Geometry check sheet. Reference: the model listing, model coordinates, mm. Face numbers are marked on the shaded views. A direction names the side the tool comes from. Coordinates: 2 decimals unless noted, no trailing zeros. Loops run counter-clockwise (first coordinate to the right, second up) from the corner with the lowest first, then second, coordinate; pieces in that order, holes last. Notation, with made-up numbers: (-29, -7) - (10, -7) arc R20 ccw to (10, 23) - close; hole circle Ø10 at (23, -11.75). An arc over 180 degrees is marked (long way). One line per item, written item: value.
Autodesk Inventor part; units mm, degrees
ref_plane "to_bolt_XY" through (3, 9.5, 0) normal (1, 0, 0) x (0, 0, -1)
ref_plane "to_bolt_YZ" through (3, 9.5, 0) normal (0, 0, -1) x (0, 1, 0)
ref_plane "to_bolt_ZX" through (3, 9.5, 0) normal (0, 1, 0) x (1, 0, 0)
sketch "_____1" plane through (0, 0, 0) normal (0, 0, 1) x (1, 0, 0)
  line L0 (-21, -15) -> (-21, -20)
  line L1 (-21, -20) -> (-7, -20)
  arc A0 (-6, -19) -> (-7, -20) centre (-6, -20) ccw
  line L2 (-6, -19) -> (6, -19)
  arc A1 (7, -20) -> (6, -19) centre (6, -20) ccw
  line L3 (7, -20) -> (21, -20)
  line L4 (21, -20) -> (21, -15)
  arc A2 (21, -15) -> (20, -14) centre (20, -15) ccw
  line L5 (20, -14) -> (10, -14)
  arc A3 (9, -13) -> (10, -14) centre (10, -13) ccw
  line L6 (9, -13) -> (9, 9)
  arc A4 (9, 9) -> (3, 15) centre (3, 9) ccw
  line L7 (3, 15) -> (-3, 15)
  arc A5 (-3, 15) -> (-9, 9) centre (-3, 9) ccw
  line L8 (-9, 9) -> (-9, -13)
  arc A6 (-10, -14) -> (-9, -13) centre (-10, -13) ccw
  line L9 (-10, -14) -> (-20, -14)
  arc A7 (-20, -14) -> (-21, -15) centre (-20, -15) ccw
extrude "Extrusion1" add sketch "_____1" along normal mid plane 11
sketch "_____2" plane through (0, 0, 0) normal (0, 0, 1) x (1, 0, 0)
  arc A0 (-1, 4.899) -> (1, 4.899) centre (0, 0) ccw
  line L0 (1, 4.899) -> (1, 35)
  line L1 (1, 35) -> (-1, 35)
  line L2 (-1, 35) -> (-1, 4.899)
extrude "Extrusion2" cut sketch "_____2" along normal mid plane 11
sketch "_____3" plane through (0, 0, 0) normal (0, 1, 0) x (1, 0, 0)
  circle A0 centre (16, 0) radius 2.75
extrude "Extrusion3" cut sketch "_____3" against normal blind 20
sketch "_____4" plane through (0, 0, 0) normal (0, 1, 0) x (1, 0, 0)
  circle A0 centre (-16, 0) radius 2.75
extrude "Extrusion4" cut sketch "_____4" against normal blind 20
sketch "_____5" plane through (0, 0, 0) normal (0, 0, 1) x (1, 0, 0)
  line L0 (50, 9.5) -> (-50, 9.5)
  line L1 (0, 9.5) -> (0, 11.65)
  line L2 (0, 11.65) -> (3, 11.65)
  line L3 (3, 11.65) -> (3, 13.5)
  line L4 (3, 13.5) -> (9, 13.5)
  line L5 (9, 13.5) -> (9, 9.5)
  line L6 (9, 9.5) -> (0, 9.5)
revolve "Revolution1" cut sketch "_____5" angle 360 about axis through (50, 9.5, 0) along (1, 0, 0)
sketch "Sketch6" plane through (-1, 4.899, 5.5) normal (1, 0, 0) x (0, 0, -1)
  point P0 (5.5, 4.601)
hole "Hole1" at (-1, 9.5, 0) direction (-1, 0, 0) diameter 3.242 depth 8 countersink diameter 4 countersink angle 90
ref_plane "to_bolt_XY" through (3, 9.5, 0) normal (1, 0, 0) x (0, 0, -1)
ref_plane "to_bolt_YZ" through (3, 9.5, 0) normal (0, 0, -1) x (0, 1, 0)
ref_plane "to_bolt_ZX" through (3, 9.5, 0) normal (0, 1, 0) x (1, 0, 0)
properties part number "C-SHA10_b"
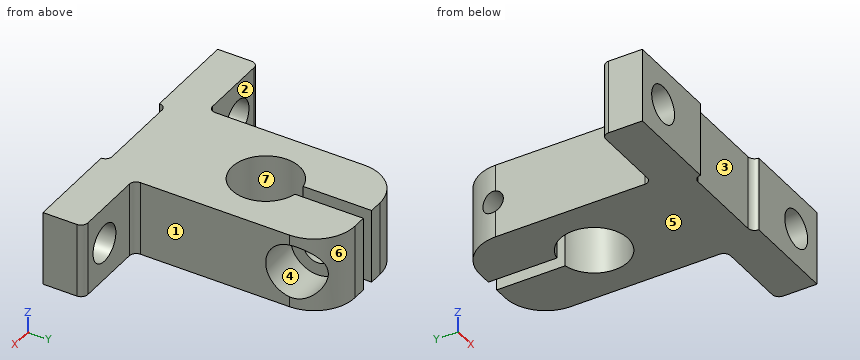
(1) Go/stop test with flat-tipped pins: pin 1 Ø5 at (x, z) = (-6, -1) entering from +Y; pin 2 Ø4 at (y, z) = (3, -2) entering from -X; pin 3 Ø3.5 at (y, z) = (9.5, 0) entering from +X; pin 4 Ø1 at (x, y) = (10, -3) entering from -Z. Record where each tip stops, or that it passes through.
Reply:
pin 1: y = 14.98
pin 2: x = -9
pin 3: x = -1.25
pin 4: through
(2) Cross-section at B-B on y = 0. Record the cut outline in (x, z), and give its area (3 significant figures).
Reply:
outline: (-9, -5.5) - (-5, -5.5) - (-5, 5.5) - (-9, 5.5) - close; (5, -5.5) - (9, -5.5) - (9, 5.5) - (5, 5.5) - close
area: 88.0 mm2
(3) Release check for a two-part mould opening along Y. For the marked faces 5, 6 and 7 record: pulls with the +Y half, pulls with the -Y half, needs draft (parallel to the pull), parting line crosses it, or undercut.
Reply:
face 5: needs draft
face 6: pulls with the +Y half
face 7: undercut
(4) Cross-section at C-C on x = -4. Record the cut outline in (y, z), and give its area (3 significant figures).
Reply:
outline: (-19, -5.5) - (-3, -5.5) - (-3, 5.5) - (-19, 5.5) - close; (3, -5.5) - (14.92, -5.5) - (14.92, 5.5) - (3, 5.5) - close; hole circle Ø3.24 at (9.5, 0)
area: 299 mm2
(5) Access from +Z, -Z, +X, -X, +Y, -Y to the whole of each face (thin tool, end or side, straight path). Record for the marked faces 1, 2, 3 and 4.
Reply:
face 1: +Z, -Z, +X, +Y
face 2: +Z, -Z, -X, +Y
face 3: +Z, -Z, -Y
face 4: +X
(6) Cross-section at A-A on x = -16. Record the cut outline in (y, z), and give its area (3 significant figures).
Reply:
outline: (-20, -5.5) - (-14, -5.5) - (-14, -2.75) - (-20, -2.75) - close; (-20, 2.75) - (-14, 2.75) - (-14, 5.5) - (-20, 5.5) - close
area: 33.0 mm2
(7) Cross-section at D-D on y = -14.5. Record the cut outline in (x, z).
Reply:
outline: (-20.87, -5.5) - (20.87, -5.5) - (20.87, 5.5) - (-20.87, 5.5) - close; hole circle Ø5.5 at (-16, 0); hole circle Ø5.5 at (16, 0)
(8) Material ranges on probe 1 along X at (y, z) = (-16.45, 0); probe 2 along Z at (x, y) = (1.95, 9.5); probe 3 along Z at (x, y) = (-8, 9.5), recorded low to high. Write a range as from..to.
Reply:
probe 1: -21..-18.75, -13.25..13.25, 18.75..21
probe 2: -5.5..-2.15, 2.15..5.5
probe 3: -5.5..-1.62, 1.62..5.5
